Part print with two shaded views. Sizes in mm from the minimum x, y, z corner. Round coordinates to 2 decimals unless told otherwise and drop trailing zeros. Loops run counter-clockwise (first coordinate to the right, second up) from the corner with the lowest first, then second, coordinate; pieces in that order, holes last. Notation, with made-up numbers: M 16.5,39 L 42.5,39 A18 ccw 42.5,71 Z; hole C -40,52 d1. An arc over 180 degrees is marked long. Put each result on its own line as item: value. Start each with the question number.
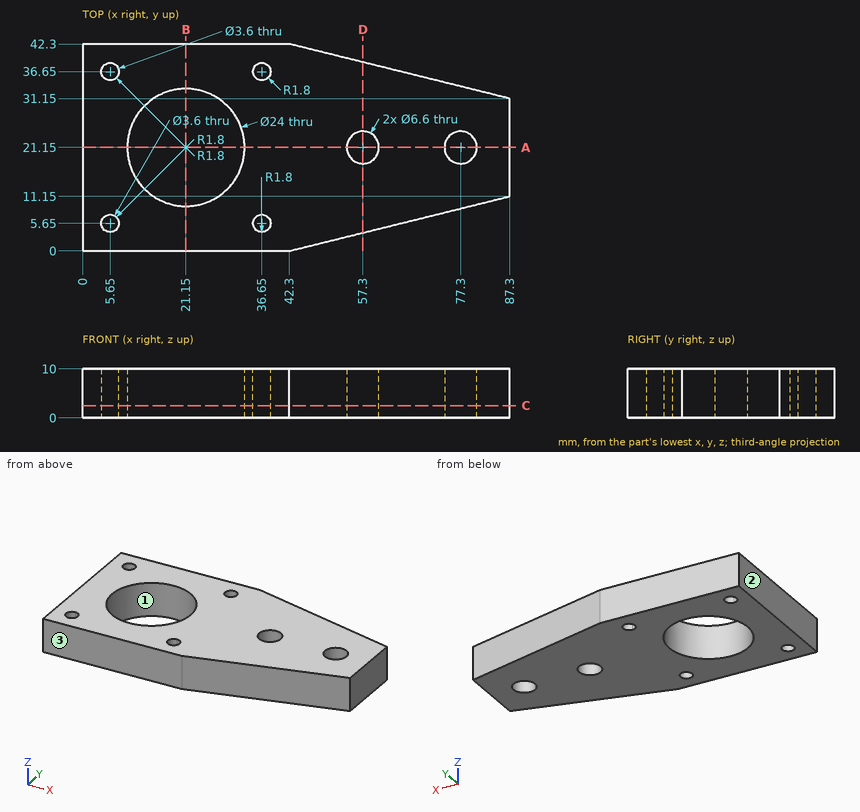
(1) Cut at A-A on y = 21.15. List the corners of the cut face in (x, z).
(2) Drill centre lines: line 1 along X through (y, z) = (21, 7.5); line 2 along X through (y, z) = (30, 3); line 3 along X through (y, z) = (13, 7). Where is each one in solid material? Low to high.
(3) Cut at C-C on z = 2.5. List the corners of the cut face in (x, y), and give its area (3 significant figures).
(4) Flat gauge pins, fed straight in: pin 1 Ø2 at (x, y) = (5.65, 5.65) entering from +Z (3 decimals); pin 2 Ø3 at (x, z) = (73.5, 8.5) entering from -Y. Where does each tip first touch, or does it go through?
(5) Cut at B-B on x = 21.15. List the corners of the cut face in (y, z), and give its area (3 significant figures).
(6) Cut at D-D on x = 57.3. List the corners of the cut face in (y, z), and give its area (3 significant figures).
(7) Mould opens along Y. For the marked faces 1, 2 and 3 say: +Y half, -Y half, draft (parallel to the pull), parting line (faces both ways), or undercut.
Taken from the geometry:
1. outline: M 0,0 L 9.15,0 L 9.15,10 L 0,10 Z; M 33.15,0 L 54,0 L 54,10 L 33.15,10 Z; M 60.6,0 L 74,0 L 74,10 L 60.6,10 Z; M 80.6,0 L 87.3,0 L 87.3,10 L 80.6,10 Z
2. line 1: 0 to 9.15, 33.15 to 54, 60.6 to 74, 80.6 to 87.3
2. line 2: 0 to 13.05, 29.25 to 87.3
2. line 3: 0 to 12.34, 29.96 to 87.3
3. outline: M 0,0 L 42.3,0 L 87.3,11.15 L 87.3,31.15 L 42.3,42.3 L 0,42.3 Z; hole C 5.65,5.65 d3.6; hole C 5.65,36.65 d3.6; hole C 21.15,21.15 d24; hole M 34.85,5.65 A1.8 ccw long 36.65,7.45 A1.8 ccw Z; hole M 36.65,34.85 A1.8 ccw 38.45,36.65 A1.8 ccw long Z; hole C 57.3,21.15 d6.6; hole C 77.3,21.15 d6.6
3. area: 2,630 mm2
4. pin 1: through
4. pin 2: y = 7.36
5. outline: M 0,0 L 9.15,0 L 9.15,10 L 0,10 Z; M 33.15,0 L 42.3,0 L 42.3,10 L 33.15,10 Z
5. area: 183 mm2
6. outline: M 3.72,0 L 17.85,0 L 17.85,10 L 3.72,10 Z; M 24.45,0 L 38.58,0 L 38.58,10 L 24.45,10 Z
6. area: 283 mm2
7. face 1: undercut
7. face 2: draft
7. face 3: -Y half
